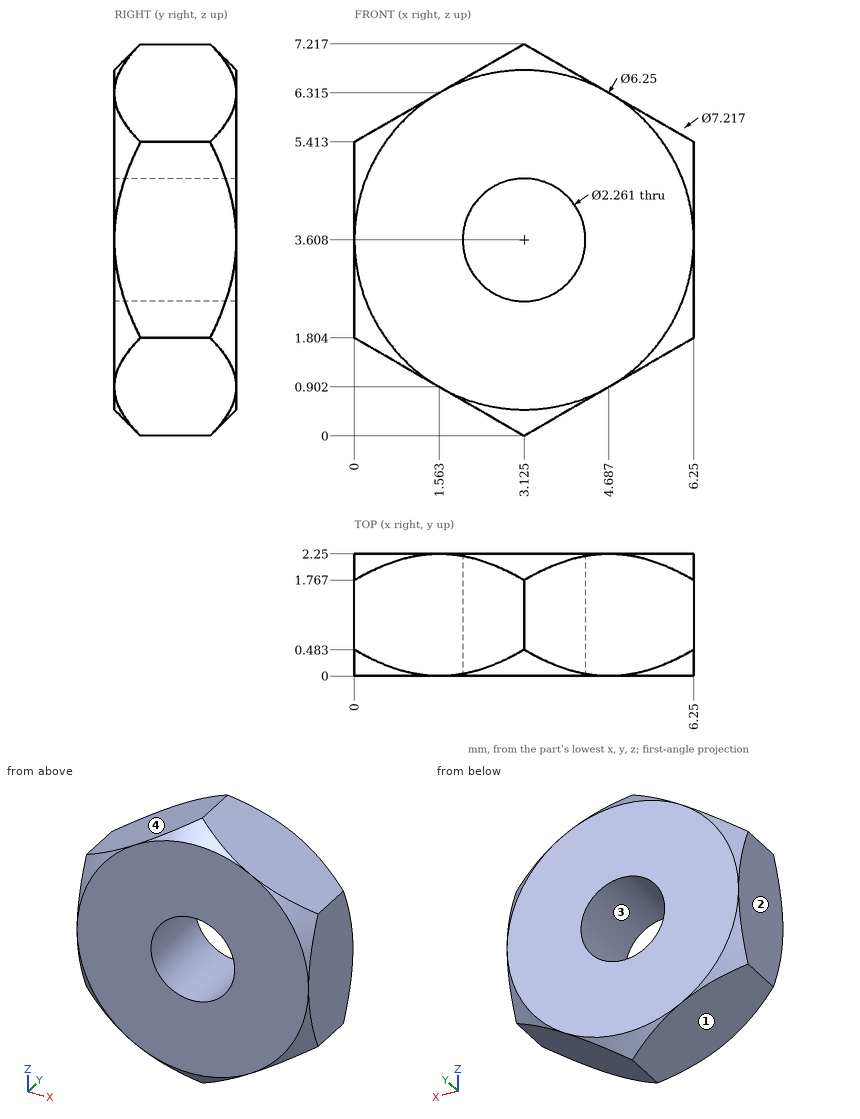
Geometry check sheet. Reference: drawing and pictorial views, mm from the part's lowest x, y, z. Give positions to 0.01 mm unless a question says otherwise; leave off trailing zeros.
1. Thickness scan on line 1 (X direction, y = 1.25, z = 3.25); line 2 (Z direction, x = 2.75, y = 0.5) (1 decimal); line 3 (X direction, y = 1.1, z = 3.5). Record the ranges inside material, lowest first.
2. Go/stop test with flat-tipped pins: pin 1 Ø1 at (y, z) = (2, 6) entering from +X (1 decimal); pin 2 Ø2 at (x, z) = (3.13, 3.61) entering from +Y. Record where each tip stops, or that it passes through.
3. Mould release check, pull along Z, two halves, no side actions. Record for the marked faces 1, 2, 3 and 4: released by +Z, released by -Z, zero draft, split by the parting line, or undercut.
Geometry says:
1. line 1: x = 0 to 2.05, 4.2 to 6.25
1. line 2: z = 0.2 to 2.5, 4.7 to 7
1. line 3: x = 0 to 2, 4.25 to 6.25
2. pin 1: stops at x = 6.1
2. pin 2: passes through
3. face 1: released by -Z
3. face 2: zero draft
3. face 3: undercut
3. face 4: released by +Z
